Build history of the part. All positions in model axes, mm. Face numbers are marked on the shaded views. Round coordinates to 2 decimals unless told otherwise and drop trailing zeros. Write item = value, one per line.
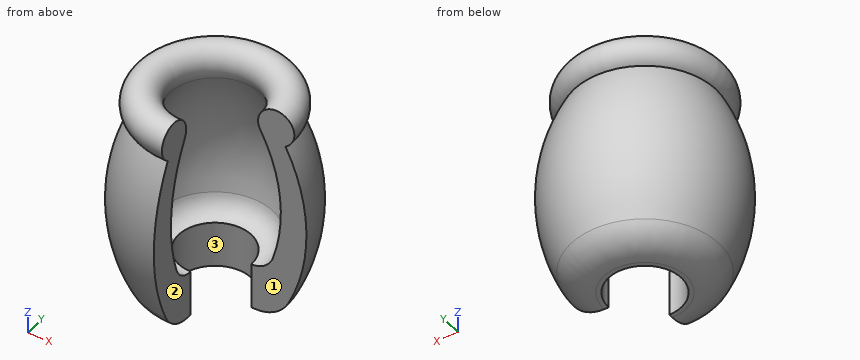
from build123d import *

# Parameters (mm, degrees)
F1_ANGLE = 270


with BuildPart() as f1:
    # F0 (on Front) → F1 (revolve)
    with BuildSketch(Plane.XZ):
        with BuildLine():
            ThreePointArc((161.981836, 170.845895), (138.910952, 139.11768), (101.6, 127))
            Line((101.6, 127), (101.6, 0))
            Line((101.6, 0), (114.3, 0))
            ThreePointArc((114.3, 0), (168.353269, 15.572073), (205.837217, 57.514879))
            ThreePointArc((205.837217, 57.514879), (256.064485, 287.322693), (197.384328, 515.118761))
            ThreePointArc((197.384328, 515.118761), (184.718228, 607.836661), (127.028262, 534.155545))
            ThreePointArc((127.028262, 534.155545), (182.331241, 356.139931), (161.981836, 170.845895))
        make_face()
    revolve(axis=Axis((0, 0, 359.91569), (0, 0, 1)), revolution_arc=F1_ANGLE)


solid = f1.part
Q1. Mould opens along Y. For the marked faces 1, 2 and 3 say: released by +Y, released by -Y, zero draft, split by the parting line, or undercut.
Check values:
face_1 = released by -Y
face_2 = zero draft
face_3 = undercut
Q2. Flat gauge pins, fed straight in: pin 1 (2 mm diameter, centred on y = 88, z = 506, fed in from -X); pin 2 (8 mm diameter, centred on x = 163.5, z = 150.5, fed in from -Y); pin 3 (2 mm diameter, centred on y = 112, z = 82.5, fed in from -X). Where does each tip first touch, or does it go through?
Check values:
pin_1 = -182.65
pin_2 = 0
pin_3 = -186.69
Q3. Probe probe 1 along Z at (x, y) = (-32, -148.5); probe 2 along Y at (x, z) = (-70, 103); probe 3 along Z at (x, y) = (-95, 38.5). List the from-to ranges inside material, lowest first.
Check values:
probe_1 = 7.22 to 151.75, 481.71 to 605.69
probe_2 = -213.92 to -73.64, 73.64 to 213.92
probe_3 = 0 to 127.01
